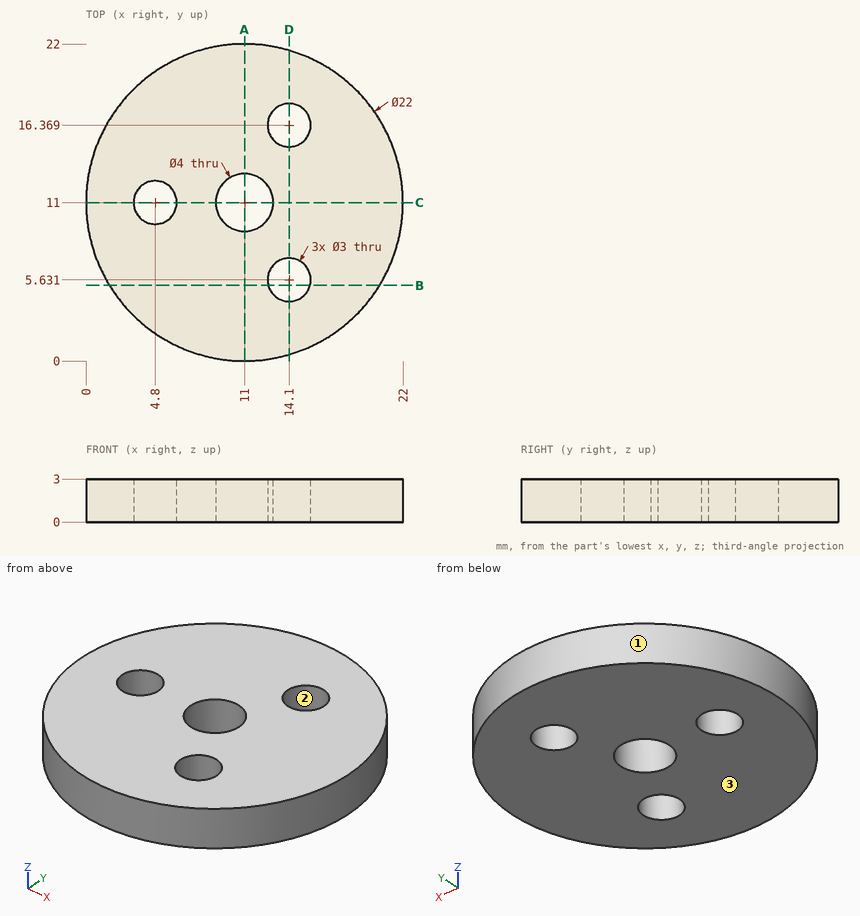
Here's the drawing with two shaded views (mm, measured from the low corner). I have some questions. Coordinates: 2 decimals unless noted, no trailing zeros. Write each loop counter-clockwise with the first axis right and the second up, starting at its lowest first coordinate (ties: lowest second). Pieces come first, ordered by that corner, then holes. Notation, with made-up numbers: (88.5, 25.25) -> (100.5, 25.25) arc R19 ccw to (100.5, 40.25) -> close; hole circle Ø9 at (-28.75, 41). An arc over 180 degrees is marked (long way). Use a Markdown table: item, result. Add a question column.
(1) We'd pull the mould along Y, two halves only. Please class the marked faces 1, 2 and 3: +Y half, -Y half, draft (parallel to the pull), parting line (faces both ways), or undercut.
(2) Please list where these lines run through material, in increasing order: line 1 (Y direction, x = 11, z = 1.5); line 2 (Y direction, x = 14.1, z = 1.5) (1 decimal); line 3 (X direction, y = 9.75, z = 1.85).
(3) If we section it at A-A, the plane x = 11: Write out the boundary of the cut face in (y, z).
(4) If we section it at C-C, the plane y = 11: Write out the boundary of the cut face in (x, z).
(5) If we section it at B-B, the plane y = 5.25: Write out the boundary of the cut face in (x, z).
(6) I'm going to push flat-ended pins straight in: P1, Ø4, axis at x = 14.1, y = 5.63, coming from the +Z side; P2, Ø2, axis at x = 14, y = 16.5, coming from the -Z side. Where does each tip first touch, or does it pass through?
(7) If we section it at D-D, the plane x = 14.1: Write out the boundary of the cut face in (y, z).
Outcome:
| question | item | result |
|---|---|---|
| 1 | face 1 | parting line |
| 1 | face 2 | undercut |
| 1 | face 3 | draft |
| 2 | line 1 | y = 0 to 9, 13 to 22 |
| 2 | line 2 | y = 0.4 to 4.1, 7.1 to 14.9, 17.9 to 21.6 |
| 2 | line 3 | x = 0.07 to 3.97, 5.63 to 9.44, 12.56 to 21.93 |
| 3 | outline | (0, 0) -> (9, 0) -> (9, 3) -> (0, 3) -> close; (13, 0) -> (22, 0) -> (22, 3) -> (13, 3) -> close |
| 4 | outline | (0, 0) -> (3.3, 0) -> (3.3, 3) -> (0, 3) -> close; (6.3, 0) -> (9, 0) -> (9, 3) -> (6.3, 3) -> close; (13, 0) -> (22, 0) -> (22, 3) -> (13, 3) -> close |
| 5 | outline | (1.62, 0) -> (12.65, 0) -> (12.65, 3) -> (1.62, 3) -> close; (15.55, 0) -> (20.38, 0) -> (20.38, 3) -> (15.55, 3) -> close |
| 6 | P1 | stops at z = 3 |
| 6 | P2 | passes through |
| 7 | outline | (0.45, 0) -> (4.13, 0) -> (4.13, 3) -> (0.45, 3) -> close; (7.13, 0) -> (14.87, 0) -> (14.87, 3) -> (7.13, 3) -> close; (17.87, 0) -> (21.55, 0) -> (21.55, 3) -> (17.87, 3) -> close |
